Geometry: final body of the model. Coordinates: model frame, mm. A direction names the side the tool comes from. Give positions to 0.01 mm unless a question says otherwise; leave off trailing zeros. Order: outer loops, then holes, each group sorted by start corner. A loop starts at its lowest first (then second) coordinate and runs counter-clockwise, first axis right, second up. Notation, with made-up numbers: M 46.25,78 L 85.25,78 A26 cw 85.25,100 Z; hole C -13.75,74 d11. An arc over 180 degrees is marked long. One line per item, written item: value. Start each with the question number.
```python
from build123d import *

# Parameters (mm, degrees)
CROQUIS1_W               = 20
CROQUIS1_H               = 46
SALIENTE_EXTRUIR1_DEPTH  = 42
CORTAR_EXTRUIR1_DEPTH    = 64.087241182
SALIENTE_EXTRUIR4_DEPTH  = 1
SALIENTE_EXTRUIR5_DEPTH  = 1
SALIENTE_EXTRUIR6_DEPTH  = 1
SALIENTE_EXTRUIR7_DEPTH  = 1
SALIENTE_EXTRUIR8_DEPTH  = 1
SALIENTE_EXTRUIR9_DEPTH  = 1
SALIENTE_EXTRUIR10_DEPTH = 1


with BuildPart() as part:
    # Croquis1 → Saliente-Extruir1 (new body)
    with BuildSketch(Plane(origin=(0, 0, 0), x_dir=(1, 0, 0), z_dir=(0, 1, 0))):
        Rectangle(CROQUIS1_W, CROQUIS1_H)
    extrude(amount=SALIENTE_EXTRUIR1_DEPTH)

    # Croquis2 → Cortar-Extruir1 (cut, through all)
    with BuildSketch(Plane.XY.offset(23)):
        Polygon((10, 0), (-0.19167841, 42.803384109), (10, 42), align=None)
    extrude(amount=-CORTAR_EXTRUIR1_DEPTH, mode=Mode.SUBTRACT)

    # Croquis3 → Saliente-Extruir4 (add, symmetric)
    with BuildSketch(Plane.XY):
        with BuildLine():
            Line((9.099065282, 3.783778611), (9.5, 3.783778611))
            ThreePointArc((9.5, 3.783778611), (9.853553391, 3.93022522), (10, 4.283778611))
            Line((10, 4.283778611), (10, 37.037089462))
            ThreePointArc((10, 37.037089462), (9.414213562, 38.451303024), (8, 39.037089462))
            Line((8, 39.037089462), (0.705093297, 39.037089462))
            Line((0.705093297, 39.037089462), (9.099065282, 3.783778611))
        make_face()
    extrude(amount=SALIENTE_EXTRUIR4_DEPTH, both=True)

    # Croquis5 → Saliente-Extruir5 (add, symmetric)
    with BuildSketch(Plane.XY.offset(6)):
        with BuildLine():
            Line((0.705093297, 39.037089462), (8, 39.037089462))
            ThreePointArc((8, 39.037089462), (9.414213562, 38.451303024), (10, 37.037089462))
            Line((10, 37.037089462), (10, 4.283778611))
            ThreePointArc((10, 4.283778611), (9.696707623, 3.768588508), (9.099065282, 3.783778611))
            Line((9.099065282, 3.783778611), (0.705093297, 39.037089462))
        make_face()
    extrude(amount=SALIENTE_EXTRUIR5_DEPTH, both=True)

    # Croquis6 → Saliente-Extruir6 (add, symmetric)
    with BuildSketch(Plane.XY.offset(11)):
        with BuildLine():
            Line((0.705093297, 39.037089462), (8, 39.037089462))
            ThreePointArc((8, 39.037089462), (9.414213562, 38.451303024), (10, 37.037089462))
            Line((10, 37.037089462), (10, 4.283778611))
            ThreePointArc((10, 4.283778611), (9.696707623, 3.768588508), (9.099065282, 3.783778611))
            Line((9.099065282, 3.783778611), (0.705093297, 39.037089462))
        make_face()
    extrude(amount=SALIENTE_EXTRUIR6_DEPTH, both=True)

    # Croquis7 → Saliente-Extruir7 (add, symmetric)
    with BuildSketch(Plane.XY.offset(16)):
        with BuildLine():
            Line((0.705093297, 39.037089462), (8, 39.037089462))
            ThreePointArc((8, 39.037089462), (9.414213562, 38.451303024), (10, 37.037089462))
            Line((10, 37.037089462), (10, 4.283778611))
            ThreePointArc((10, 4.283778611), (9.251976893, 3.716372197), (8.907184659, 4.589645878))
            Line((8.907184659, 4.589645878), (0.705093297, 39.037089462))
        make_face()
    extrude(amount=SALIENTE_EXTRUIR7_DEPTH, both=True)

    # Croquis9 → Saliente-Extruir8 (add, symmetric)
    with BuildSketch(Plane(origin=(0, 0, -6), x_dir=(-1, 0, 0), z_dir=(0, 0, -1))):
        with BuildLine():
            Line((-0.705093297, 39.037089462), (-8, 39.037089462))
            ThreePointArc((-8, 39.037089462), (-9.414213562, 38.451303024), (-10, 37.037089462))
            Line((-10, 37.037089462), (-10, 4.283778611))
            ThreePointArc((-10, 4.283778611), (-9.696707623, 3.768588508), (-9.099065282, 3.783778611))
            Line((-9.099065282, 3.783778611), (-0.705093297, 39.037089462))
        make_face()
    extrude(amount=SALIENTE_EXTRUIR8_DEPTH, both=True)

    # Croquis10 → Saliente-Extruir9 (add, symmetric)
    with BuildSketch(Plane(origin=(0, 0, -11), x_dir=(-1, 0, 0), z_dir=(0, 0, -1))):
        with BuildLine():
            Line((-0.705093297, 39.037089462), (-8, 39.037089462))
            ThreePointArc((-8, 39.037089462), (-9.414213562, 38.451303024), (-10, 37.037089462))
            Line((-10, 37.037089462), (-10, 4.283778611))
            ThreePointArc((-10, 4.283778611), (-9.696707623, 3.768588508), (-9.099065282, 3.783778611))
            Line((-9.099065282, 3.783778611), (-8.907184659, 4.589645878))
            Line((-8.907184659, 4.589645878), (-0.705093297, 39.037089462))
        make_face()
    extrude(amount=SALIENTE_EXTRUIR9_DEPTH, both=True)

    # Croquis11 → Saliente-Extruir10 (add, symmetric)
    with BuildSketch(Plane(origin=(0, 0, -16), x_dir=(-1, 0, 0), z_dir=(0, 0, -1))):
        with BuildLine():
            Line((-0.705093297, 39.037089462), (-8, 39.037089462))
            ThreePointArc((-8, 39.037089462), (-9.414213562, 38.451303024), (-10, 37.037089462))
            Line((-10, 37.037089462), (-10, 4.283778611))
            ThreePointArc((-10, 4.283778611), (-9.696707623, 3.768588508), (-9.099065282, 3.783778611))
            Line((-9.099065282, 3.783778611), (-0.705093297, 39.037089462))
        make_face()
    extrude(amount=SALIENTE_EXTRUIR10_DEPTH, both=True)


solid = part.part
```
Q1. Contact query for flat-ended pins moving along their axis: pin 1 (7.5 mm diameter, centred on x = 7, y = 27, fed in from -Z); pin 2 (0.6 mm diameter, centred on x = 4, z = 0.5, fed in from +Y). Output: stop coordinate, or through.
Q2. Ray query, line 1 along Y through (x, z) = (1, -6); line 2 along X through (y, z) = (18, -8); line 3 along X through (y, z) = (10, 13.5). Return the intervals inside material, ascending. Write a range as [from, to].
Q3. Set-up query: faces 1 (the face through (6, 26, -5)), 2 (the face through (0, 0, 0)), 3 (the face through (6, 26, 17)), 4 (the face through (4, 39.037, 6)). Return all of +Z, -Z, +X, -X, +Y, -Y with unobstructed straight access to the full face (end or side cutting, diameter ignored); none if empty.
Q4. Section query C-C on z = 3. Return loops of the section in (x, y), and give its area (3 significant figures).
Results below:
1. pin 1: z = -23
1. pin 2: y = 39.04
2. line 1: [0, 39.04]
2. line 2: [-10, 5.71]
2. line 3: [-10, 7.62]
3. face 1: +X, +Y
3. face 2: +Z, -Z, +X, -X, -Y
3. face 3: +Z, +X, +Y
3. face 4: +Z, -Z, +X, +Y
4. outline: M -10,0 L 10,0 L 0,42 L -10,42 Z
4. area: 630 mm2
